Geometry check sheet. Reference: the model listing, model coordinates, mm. Coordinates: 2 decimals unless noted, no trailing zeros. Write each loop counter-clockwise with the first axis right and the second up, starting at its lowest first coordinate (ties: lowest second). Pieces come first, ordered by that corner, then holes. Notation, with made-up numbers: M 45.25,10.25 L 57.25,10.25 A21 cw 57.25,16.25 Z; hole C 21.25,38 d7. An arc over 180 degrees is marked long. Answer as a JSON object with one key per item and string values. Group by question number.
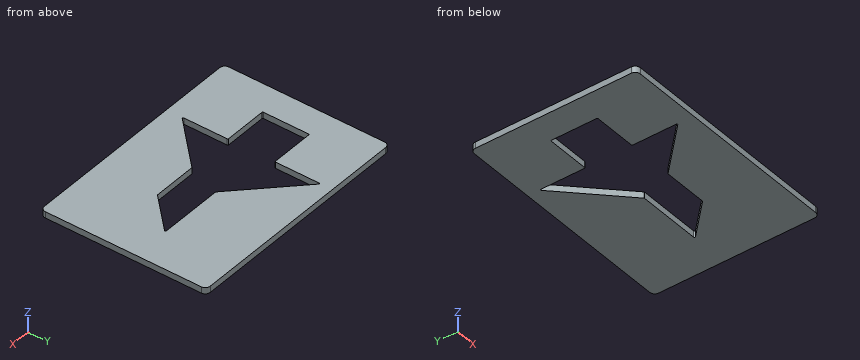
```python
from build123d import *

# Parameters (mm, degrees)
F1_DEPTH = 6.35
F3_DEPTH = 6.351
F5_DEPTH = 6.351


with BuildPart() as f1:
    # F0 (on Top) → F1 (new body)
    with BuildSketch(Plane.XY):
        with BuildLine():
            Line((113.9825, 84.1375), (-113.9825, 84.1375))
            ThreePointArc((-113.9825, 84.1375), (-117.574602, 82.649602), (-119.0625, 79.0575))
            Line((-119.0625, 79.0575), (-119.0625, -79.0575))
            ThreePointArc((-119.0625, -79.0575), (-117.574602, -82.649602), (-113.9825, -84.1375))
            Line((-113.9825, -84.1375), (113.9825, -84.1375))
            ThreePointArc((113.9825, -84.1375), (117.574602, -82.649602), (119.0625, -79.0575))
            Line((119.0625, -79.0575), (119.0625, 79.0575))
            ThreePointArc((119.0625, 79.0575), (117.574602, 82.649602), (113.9825, 84.1375))
        make_face()
    extrude(amount=F1_DEPTH)

    # F2 (on face) → F3 (cut, through all)
    with BuildSketch(Plane.XY.offset(6.35)):
        Polygon((-88.5825, 24.343994), (-88.5825, -20.614006), (-43.6245, -20.614006), (-43.6245, -65.538781), (1.276781, -20.6375), (46.234781, -20.6375), (78.024887, 11.152607), (14.524887, 11.152607), (-43.6245, 69.301994), (-43.6245, 24.343994), align=None)
    extrude(amount=-F3_DEPTH, mode=Mode.SUBTRACT)

    # F4 (on face) → F5 (cut, through all)
    with BuildSketch(Plane.XY.offset(6.35)):
        with BuildLine():
            ThreePointArc((79.746763, 11.078431), (79.917449, 11.936532), (79.189987, 12.422607))
            Line((79.189987, 12.422607), (15.37709, 12.422607))
            ThreePointArc((15.37709, 12.422607), (15.075765, 12.482544), (14.820314, 12.653231))
            Line((14.820314, 12.653231), (-43.550324, 71.023869))
            ThreePointArc((-43.550324, 71.023869), (-44.408425, 71.194556), (-44.8945, 70.467093))
            Line((-44.8945, 70.467093), (-44.8945, 26.401394))
            ThreePointArc((-44.8945, 26.401394), (-45.125124, 25.844618), (-45.6819, 25.613994))
            Line((-45.6819, 25.613994), (-89.0651, 25.613994))
            ThreePointArc((-89.0651, 25.613994), (-89.621876, 25.38337), (-89.8525, 24.826594))
            Line((-89.8525, 24.826594), (-89.8525, -21.096606))
            ThreePointArc((-89.8525, -21.096606), (-89.621876, -21.653382), (-89.0651, -21.884006))
            Line((-89.0651, -21.884006), (-45.6819, -21.884006))
            ThreePointArc((-45.6819, -21.884006), (-45.125124, -22.11463), (-44.8945, -22.671406))
            Line((-44.8945, -22.671406), (-44.8945, -66.70388))
            ThreePointArc((-44.8945, -66.70388), (-44.408425, -67.431343), (-43.550324, -67.260656))
            Line((-43.550324, -67.260656), (1.572208, -22.138124))
            ThreePointArc((1.572208, -22.138124), (1.827659, -21.967437), (2.128984, -21.9075))
            Line((2.128984, -21.9075), (46.43468, -21.9075))
            ThreePointArc((46.43468, -21.9075), (46.736005, -21.847563), (46.991456, -21.676876))
            Line((46.991456, -21.676876), (79.746763, 11.078431))
        make_face()
    extrude(amount=-F5_DEPTH, mode=Mode.SUBTRACT)


solid = f1.part
```
1) Section check B-B (x = 22.5). Record the cut outline in (y, z).
2) Section check C-C (y = -4.5). Record the cut outline in (x, z).
3) Material ranges on probe 1 along Y at (x, z) = (-88, 6.25); probe 2 along Y at (x, z) = (28.5, 0.75); probe 3 along X at (y, z) = (-33.5, 3), recorded low to high. Write a range as [from, to].
4) Section check A-A (z = 1.75). Record the cut outline in (x, y), then the cut area to 3 significant figures.
Entries:
{
 "1": {"outline": "M -84.14,0 L -21.91,0 L -21.91,6.35 L -84.14,6.35 Z; M 12.42,0 L 84.14,0 L 84.14,6.35 L 12.42,6.35 Z"},
 "2": {"outline": "M -119.06,0 L -89.85,0 L -89.85,6.35 L -119.06,6.35 Z; M 64.17,0 L 119.06,0 L 119.06,6.35 L 64.17,6.35 Z"},
 "3": {"probe 1": "[-84.14, -21.88], [25.61, 84.14]", "probe 2": "[-84.14, -21.91], [12.42, 84.14]", "probe 3": "[-119.06, -44.89], [-9.79, 119.06]"},
 "4": {"outline": "M -119.06,-79.06 A5.08 ccw -113.98,-84.14 L 113.98,-84.14 A5.08 ccw 119.06,-79.06 L 119.06,79.06 A5.08 ccw 113.98,84.14 L -113.98,84.14 A5.08 ccw -119.06,79.06 Z; hole M -89.85,-21.1 A0.79 ccw -89.07,-21.88 L -45.68,-21.88 A0.79 cw -44.89,-22.67 L -44.89,-66.7 A0.79 ccw -43.55,-67.26 L 1.57,-22.14 A0.79 cw 2.13,-21.91 L 46.43,-21.91 A0.79 ccw 46.99,-21.68 L 79.75,11.08 A0.79 ccw 79.19,12.42 L 15.38,12.42 A0.79 cw 14.82,12.65 L -43.55,71.02 A0.79 ccw -44.89,70.47 L -44.89,26.4 A0.79 cw -45.68,25.61 L -89.07,25.61 A0.79 ccw -89.85,24.83 Z", "area": "31,300 mm^2"}
}
